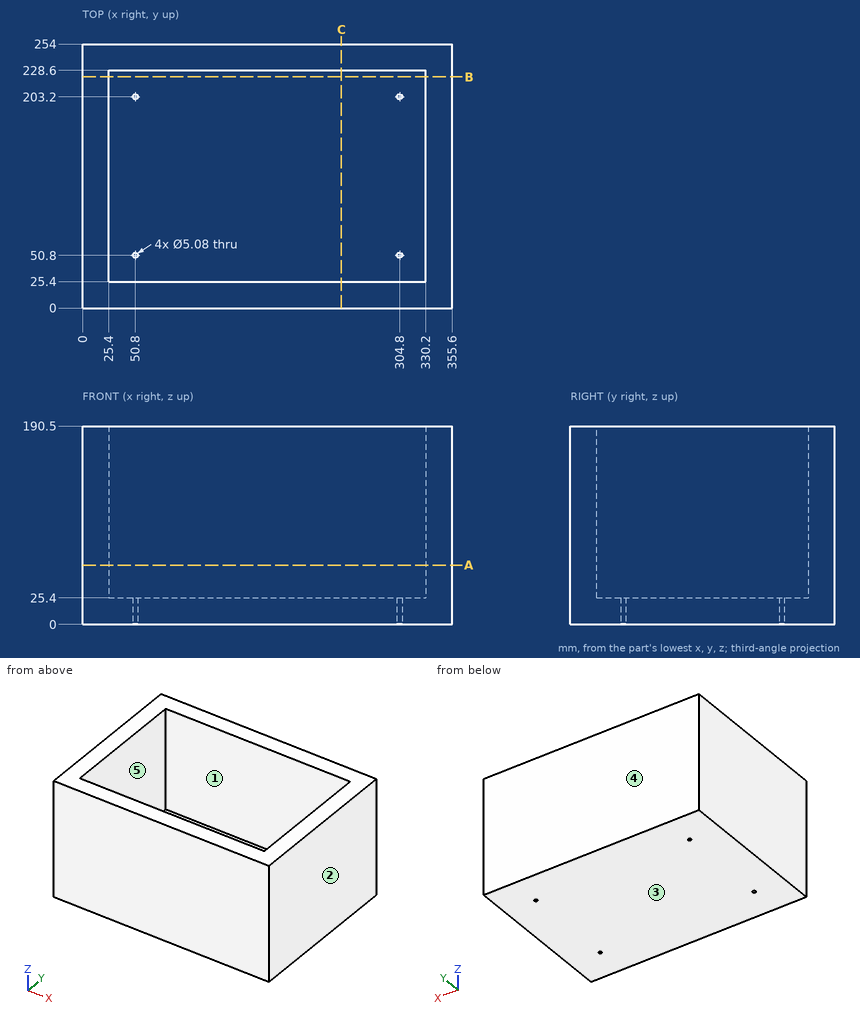
Geometry: see drawing. Coordinates: mm, zero at the bounding-box minimum. A direction names the side the tool comes from. Coordinates: 2 decimals unless noted, no trailing zeros. Write each loop counter-clockwise with the first axis right and the second up, starting at its lowest first coordinate (ties: lowest second). Pieces come first, ordered by that corner, then holes. Notation, with made-up numbers: M 86.25,19 L 120.25,19 A34 cw 120.25,50 Z; hole C 1,-31.5 d2. An arc over 180 degrees is marked long. Answer as a JSON object with one key per item and string values.
1. Ray query, L1, parallel to Y at x = 50.8, z = 6.75; L2, parallel to X at y = 203.2, z = 13.25; L3, parallel to X at y = 200, z = 140.5. Return the intervals inside material, ascending.
Evaluation:
{"L1": "0 to 48.26, 53.34 to 200.66, 205.74 to 254", "L2": "0 to 48.26, 53.34 to 302.26, 307.34 to 355.6", "L3": "0 to 25.4, 330.2 to 355.6"}
2. Cut plane B-B on y = 222.5. Output: boundary loops of the cut face in (x, z), plus the area to 3 significant figures.
Evaluation:
{"outline": "M 0,0 L 355.6,0 L 355.6,190.5 L 330.2,190.5 L 330.2,25.4 L 25.4,25.4 L 25.4,190.5 L 0,190.5 Z", "area": "17,400 mm^2"}
3. Cut plane A-A on z = 57. Output: boundary loops of the cut face in (x, y).
Evaluation:
{"outline": "M 0,0 L 355.6,0 L 355.6,254 L 0,254 Z; hole M 25.4,25.4 L 330.2,25.4 L 330.2,228.6 L 25.4,228.6 Z"}
4. Contact query for flat-ended pins moving along their axis: P1, Ø4.5, axis at x = 50.8, y = 50.8, coming from the -Z side; P2, Ø8, axis at x = 304.8, y = 203.2, coming from the +Z side. Output: stop coordinate, or through.
Evaluation:
{"P1": "through", "P2": "z = 25.4"}
5. Access query for the marked faces 1 and 2. Directions: +Z, -Z, +X, -X, +Y, -Y. A direction counts if a zero-diameter tool reaches every point of the face in a straight line with its end or side. Return the directions, or none.
Evaluation:
{"face 1": "+Z", "face 2": "+Z, -Z, +X, +Y, -Y"}
6. Draft query along Y for the marked faces 3, 4 and 5. Return one class per face: released by +Y, released by -Y, zero draft, split by the parting line, or undercut.
Evaluation:
{"face 3": "zero draft", "face 4": "released by +Y", "face 5": "undercut"}
7. Cut plane C-C on x = 249. Output: boundary loops of the cut face in (y, z), plus the area to 3 significant figures.
Evaluation:
{"outline": "M 0,0 L 254,0 L 254,190.5 L 228.6,190.5 L 228.6,25.4 L 25.4,25.4 L 25.4,190.5 L 0,190.5 Z", "area": "14,800 mm^2"}
